Input: part model. Units: mm. Frame: model coordinates. A direction names the side the tool comes from. Give positions to 0.01 mm unless a question says otherwise; leave off trailing zeros. Write each loop counter-clockwise with the first axis right and the second up, starting at its lowest first coordinate (ties: lowest second). Pieces come first, ordered by that corner, then holes.
```python
from build123d import *

# Parameters (mm, degrees)
F1_DEPTH = 25.4
F2_R     = 15.1511
F3_DEPTH = 71.374
F4_DEPTH = 28.448
F5_R     = 5.08


with BuildPart() as f1:
    # F0 (on Front) → F1 (new body)
    with BuildSketch(Plane.XZ):
        with BuildLine():
            ThreePointArc((-106.8790640436, -27.94), (-87.1225005772, -19.7565634664), (-78.9390640436, 0))
            ThreePointArc((-78.9390640436, 0), (-87.1225005772, 19.7565634664), (-106.8790640436, 27.94))
            ThreePointArc((-106.8790640436, 27.94), (-134.8190640436, 0), (-106.8790640436, -27.94))
        make_face()
        with BuildLine():
            ThreePointArc((-106.8790640436, 27.94), (-87.1225005772, 19.7565634664), (-78.9390640436, 0))
            ThreePointArc((-78.9390640436, 0), (-87.1225005772, -19.7565634664), (-106.8790640436, -27.94))
            Line((-106.8790640436, -27.94), (60.9095794208, -27.94))
            ThreePointArc((60.9095794208, -27.94), (32.9695794208, 0), (60.9095794208, 27.94))
            Line((60.9095794208, 27.94), (-106.8790640436, 27.94))
        make_face()
        with BuildLine():
            ThreePointArc((88.8495794208, 0), (80.6661428872, 19.7565634664), (60.9095794208, 27.94))
            ThreePointArc((60.9095794208, 27.94), (32.9695794208, 0), (60.9095794208, -27.94))
            ThreePointArc((60.9095794208, -27.94), (80.6661428872, -19.7565634664), (88.8495794208, 0))
        make_face()
    extrude(amount=F1_DEPTH)

    # F2 (on Front) → F3 (join)
    with BuildSketch(Plane.XZ):
        with Locations((62.2427165988, 0)):
            Circle(F2_R)
    extrude(amount=F3_DEPTH)

    # F4 (add): a face of the model
    f4_faces = [f1.faces().sort_by_distance(p)[0] for p in [
        (62.2427165988, -71.374, 0),
    ]]
    extrude(f4_faces, amount=F4_DEPTH)

    # F5
    f5_edges = [f1.edges().sort_by_distance(p)[0] for p in [
        (-22.984742, 0, 27.94),
        (-134.819064, -25.4, 0),
        (47.091617, -99.822, 0),
    ]]
    fillet(f5_edges, radius=F5_R)


solid = f1.part
```
Q1. Section B-B, the plane y = -31. Return the cut outline in (x, z), then the cut area to 3 significant figures.
Q2. Material intervals for line 1 along Y through (x, z) = (-2, -4.5); line 2 along X through (y, z) = (-44, 0); line 3 along Z through (x, y) = (63, -13.5), sorted ascending.
Q3. Section C-C, the plane y = -16. Return the cut outline in (x, z), then the cut area to 3 significant figures.
Q4. Section A-A, the plane x = -102.5. Return the cut outline in (y, z), then the cut area to 3 significant figures.
Q5. Access query for faces 1 (the cylindrical face through (50.22, -59.59, -9.22)), 2 (the cylindrical face through (-134.812, -12.593, 0.614)). Directions: +Z, -Z, +X, -X, +Y, -Y. A direction counts if a zero-diameter tool reaches every point of the face in a straight line with its end or side. Return the directions, or none.
Q6. Pin query (flat end, axial travel): pin 1 (6 mm diameter, centred on x = 38, z = 18, fed in from -Y); pin 2 (3 mm diameter, centred on x = 61, y = -64, fed in from +Z). Return the tip coordinate at first contact, or that it passes through.
Solutions:
1. outline: circle Ø30.3 at (62.24, 0)
1. area: 721 mm2
2. line 1: y = -25.4 to 0
2. line 2: x = 47.09 to 77.39
2. line 3: z = -27.86 to 27.86
3. outline: (-106.88, -27.94) - (60.91, -27.94) arc R27.94 ccw to (60.91, 27.94) - (-106.88, 27.94) arc R27.94 ccw to start
3. area: 11,800 mm2
4. outline: (-25.4, -22.86) arc R5.08 ccw to (-20.32, -27.94) - (-5.08, -27.94) arc R5.08 ccw to (0, -22.86) - (0, 22.86) arc R5.08 ccw to (-5.08, 27.94) - (-20.32, 27.94) arc R5.08 ccw to (-25.4, 22.86) - close
4. area: 1,400 mm2
5. face 1: -Y
5. face 2: -X, +Y, -Y
6. pin 1: stops at y = -25.4
6. pin 2: stops at z = 15.15
